```python
from build123d import *

# Parameters (mm, degrees)
SKETCH2_R                = 4
BOSS_EXTRUDE1_DEPTH      = 25
SHELL1_START             = 4
SHELL1_DEPTH             = 17
SKETCH4_W                = 10
SKETCH4_H                = 16
CUT_EXTRUDE1_DEPTH       = 2
SKETCH5_W                = 10
SKETCH5_H                = 16
CUT_EXTRUDE2_DEPTH       = 2
BOSS_EXTRUDE2_REACH      = 60.764
BOSS_EXTRUDE2_END_RADIUS = 34.587437562
SKETCH12_W               = 3
SKETCH12_H               = 2
CUT_EXTRUDE3_DEPTH       = 16
FILLET1_R                = 5
SKETCH14_R               = 8
CUT_EXTRUDE4_DEPTH       = 17


# Read off the part's stored shape, not the designer's step: Shell1
with BuildPart() as part:
    # Sketch2 → Boss-Extrude1 (new body)
    with BuildSketch(Plane.XY):
        with BuildLine():
            ThreePointArc((-16.302119642, 29.796788513), (8.090433332, 34.669313021), (30.38825142, 23.64454798))
            ThreePointArc((30.38825142, 23.64454798), (31.608808708, 19.602540573), (29.864628369, 15.757359313))
            Line((29.864628369, 15.757359313), (14.107269056, 0))
            Line((14.107269056, 0), (-10.892730944, 0))
            Line((-10.892730944, 0), (-23.748483138, 15.320888862))
            Line((-23.748483138, 15.320888862), (-40.039838772, 20.178020896))
            Line((-40.039838772, 20.178020896), (-37.182702282, 29.761171269))
            Line((-37.182702282, 29.761171269), (-18.016401536, 24.046898289))
            Line((-18.016401536, 24.046898289), (-16.302119642, 29.796788513))
        make_face()
        with Locations((25.621987682, 20)):
            Circle(SKETCH2_R, mode=Mode.SUBTRACT)
    extrude(amount=BOSS_EXTRUDE1_DEPTH)

    # Shell1 outline → Shell1 (cut)
    with BuildSketch(Plane.XY.offset(SHELL1_START)):
        with BuildLine():
            ThreePointArc((20.592180868, 26.221016269), (3.939176513, 30.988554812), (-12.936984293, 27.083791792))
            Line((-12.936984293, 27.083791792), (-15.325995982, 19.070783543))
            Line((-15.325995982, 19.070783543), (-34.492296729, 24.785056524))
            Line((-34.492296729, 24.785056524), (-36.206578623, 19.0351663))
            Line((-36.206578623, 19.0351663), (-23.748483138, 15.320888862))
            Line((-23.748483138, 15.320888862), (-10.892730944, 0))
            Line((-10.892730944, 0), (14.107269056, 0))
            Line((14.107269056, 0), (26.122970982, 12.015701926))
            ThreePointArc((26.122970982, 12.015701926), (18.16710341, 17.097466537), (20.592180868, 26.221016269))
        make_face()
    extrude(amount=SHELL1_DEPTH, mode=Mode.SUBTRACT)

    # Sketch4 → Cut-Extrude1 (cut)
    with BuildSketch(Plane.XY.offset(4)):
        with Locations((1.107269056, 8)):
            Rectangle(SKETCH4_W, SKETCH4_H)
    extrude(amount=-CUT_EXTRUDE1_DEPTH, mode=Mode.SUBTRACT)

    # Sketch5 → Cut-Extrude2 (cut)
    with BuildSketch(Plane(origin=(0, 0, 21), x_dir=(-1, 0, 0), z_dir=(0, 0, -1))):
        with Locations((-1.107269056, 8)):
            Rectangle(SKETCH5_W, SKETCH5_H)
    extrude(amount=-CUT_EXTRUDE2_DEPTH, mode=Mode.SUBTRACT)

    # Boss-Extrude2: up to this cylinder (the profile starts inside it)
    boss_extrude2_end = Plane(origin=(3.049463937, -3.587437562, 12.5), z_dir=(0, 0, -1)) * Cylinder(BOSS_EXTRUDE2_END_RADIUS, 206.702875123, mode=Mode.PRIVATE)
    # Sketch12 → Boss-Extrude2 (add, up to the surface)
    with BuildSketch(Plane.XZ, mode=Mode.PRIVATE) as boss_extrude2_sk1:
        with Locations((-5.392730944, 20)):
            Rectangle(SKETCH12_W, SKETCH12_H)
    boss_extrude2_tool1 = extrude(boss_extrude2_sk1.sketch, amount=-BOSS_EXTRUDE2_REACH, mode=Mode.PRIVATE) & boss_extrude2_end
    add(boss_extrude2_tool1.solids().sort_by_distance((-5.392731, 0, 20))[0])
    # Sketch12 → Boss-Extrude2 (add, up to the surface)
    with BuildSketch(Plane.XZ, mode=Mode.PRIVATE) as boss_extrude2_sk2:
        with Locations((7.607269056, 20)):
            Rectangle(SKETCH12_W, SKETCH12_H)
    boss_extrude2_tool2 = extrude(boss_extrude2_sk2.sketch, amount=-BOSS_EXTRUDE2_REACH, mode=Mode.PRIVATE) & boss_extrude2_end
    add(boss_extrude2_tool2.solids().sort_by_distance((7.607269, 0, 20))[0])
    # Sketch12 → Boss-Extrude2 (add, up to the surface)
    with BuildSketch(Plane.XZ, mode=Mode.PRIVATE) as boss_extrude2_sk3:
        with Locations((-5.392730944, 5)):
            Rectangle(SKETCH12_W, SKETCH12_H)
    boss_extrude2_tool3 = extrude(boss_extrude2_sk3.sketch, amount=-BOSS_EXTRUDE2_REACH, mode=Mode.PRIVATE) & boss_extrude2_end
    add(boss_extrude2_tool3.solids().sort_by_distance((-5.392731, 0, 5))[0])
    # Sketch12 → Boss-Extrude2 (add, up to the surface)
    with BuildSketch(Plane.XZ, mode=Mode.PRIVATE) as boss_extrude2_sk4:
        with Locations((7.607269056, 5)):
            Rectangle(SKETCH12_W, SKETCH12_H)
    boss_extrude2_tool4 = extrude(boss_extrude2_sk4.sketch, amount=-BOSS_EXTRUDE2_REACH, mode=Mode.PRIVATE) & boss_extrude2_end
    add(boss_extrude2_tool4.solids().sort_by_distance((7.607269, 0, 5))[0])

    # Sketch13 → Cut-Extrude3 (cut)
    with BuildSketch(Plane.XY.offset(25)):
        Polygon((-32.391127096, 28.332603024), (-35.248263586, 18.749452651), (-28.540058324, 16.749457107), (-25.682921834, 26.332607481), align=None)
    extrude(amount=-CUT_EXTRUDE3_DEPTH, mode=Mode.SUBTRACT)

    # Fillet1
    fillet1_edges = [part.edges().sort_by_distance(p)[0] for p in [
        (-34.786914689, 29.046887146, 25),
        (-21.849661685, 25.189752885, 25),
    ]]
    fillet(fillet1_edges, radius=FILLET1_R)

    # Sketch14 → Cut-Extrude4 (cut)
    with BuildSketch(Plane.XY.offset(4)):
        with Locations((25.621987682, 20)):
            Circle(SKETCH14_R)
    extrude(amount=CUT_EXTRUDE4_DEPTH, mode=Mode.SUBTRACT)


solid = part.part
```
Can you work these out from the model? Positions are in its coordinate system, mm. A direction names the side the tool comes from. Coordinates: 2 decimals unless noted, no trailing zeros. Loops run counter-clockwise (first coordinate to the right, second up) from the corner with the lowest first, then second, coordinate; pieces in that order, holes last. Notation, with made-up numbers: (-11, 16) -> (16, 16) arc R19 cw to (16, 41) -> close; hole circle Ø1 at (44.5, -33). An arc over 180 degrees is marked (long way). Answer as a JSON object with one key per item and string values.
1) If I drill on line 1 (Z direction, x = -19, y = 19.5); line 2 (Z direction, x = 1.5, y = 2.5); line 3 (Y direction, x = -5, z = 18.75), over which ranges is the centre line in solid material (lowest first)?
Results:
{"line 1": "z = 0 to 4, 21 to 25", "line 2": "z = 0 to 2, 23 to 25", "line 3": "y = 30.05 to 34.15"}
2) For P1, Ø1.2, axis at y = 18.5, z = 3, coming from the +X side; P2, Ø10, axis at y = 17, z = 12.5, coming from the +X side; P3, Ø3, axis at x = -9, z = 15.5, coming from the +Y side, each with a flat end and sliding along its axis, tell me the tip position at first contact or that it passes through.
Results:
{"P1": "stops at x = 31.55", "P2": "stops at x = -14.45", "P3": "stops at y = 33.53"}
3) For faces 1 (the face through (-6.893, 15, 20)), 2 (the face through (-26.497, 23.604, 18.89)), 3 (the face through (-33.482, 24.673, 18.89)), 4 (the face through (22.67, 22.7, 22.97)), which set-ups out of +Z, -Z, +X, -X, +Y, -Y let a thin tool reach every point of the face, with its end or its side?
Results:
{"face 1": "-Y", "face 2": "+Z, +Y", "face 3": "+Z, -Y", "face 4": "+Z, -Z"}
4) Imagine slicing it at B-B (z = 3.25). Please give me the cut outline in (x, y).
Results:
{"outline": "(-40.04, 20.18) -> (-23.75, 15.32) -> (-10.89, 0) -> (-3.89, 0) -> (-3.89, 16) -> (6.11, 16) -> (6.11, 0) -> (14.11, 0) -> (29.86, 15.76) arc R6 ccw to (30.39, 23.64) arc R38.59 ccw to (-16.3, 29.8) -> (-18.02, 24.05) -> (-37.18, 29.76) -> close; hole circle Ø8 at (25.62, 20)"}
5) Thinking about a two-plate mould opening in X: for faces 5 (the face through (-3.893, 12, 21)), 6 (the face through (-37.211, 19.334, 9.547)), 7 (the face through (1.4, 0, 1.7)), which applies, pulls with the +X half, pulls with the -X half, needs draft (parallel to the pull), parting line crosses it, or undercut?
Results:
{"face 5": "undercut", "face 6": "pulls with the -X half", "face 7": "needs draft"}
6) Imagine slicing it at D-D (x = 7.5). Please give me the cut outline in (y, z), then the cut area to 3 significant figures.
Results:
{"outline": "(0, 0) -> (34.74, 0) -> (34.74, 25) -> (0, 25) -> (0, 19) -> (30.71, 19) -> (30.71, 6) -> (0, 6) -> close", "area": "469 mm^2"}
7) Imagine slicing it at C-C (z = 12.5). Please give me the cut outline in (x, y).
Results:
{"outline": "(-40.04, 20.18) -> (-36.21, 19.04) -> (-34.49, 24.79) -> (-33.53, 24.5) -> (-32.39, 28.33) -> (-37.18, 29.76) -> close; (-26.83, 22.5) -> (-15.33, 19.07) -> (-12.94, 27.08) arc R34.59 cw to (20.59, 26.22) arc R8 cw to (25.23, 27.99) arc R38.59 ccw to (-16.3, 29.8) -> (-18.02, 24.05) -> (-25.68, 26.33) -> close"}
8) Imagine slicing it at A-A (y = 13.5). Please give me the cut outline in (x, z).
Results:
{"outline": "(-22.22, 0) -> (27.61, 0) -> (27.61, 4) -> (9.11, 4) -> (9.11, 6) -> (6.11, 6) -> (6.11, 2) -> (-3.89, 2) -> (-3.89, 6) -> (-6.89, 6) -> (-6.89, 4) -> (-22.22, 4) -> close; (-22.22, 21) -> (-6.89, 21) -> (-6.89, 19) -> (-3.89, 19) -> (-3.89, 23) -> (6.11, 23) -> (6.11, 19) -> (9.11, 19) -> (9.11, 21) -> (27.61, 21) -> (27.61, 25) -> (-22.22, 25) -> close"}
